from build123d import *

# Parameters (mm, degrees)
F2_DEPTH = 6
F3_R     = 1.5
F6_R     = 1.75
F7_DEPTH = 9
F8_R     = 3.5
F9_DEPTH = 5


with BuildPart() as f2:
    # F1 (on Front) → F2 (new body, symmetric)
    with BuildSketch(Plane.XZ):
        Polygon((-9, 0), (0, 0), (0, 70), (6, 70), (6, 66), (30, 66), (30, 79), (-9, 79), align=None)
    extrude(amount=F2_DEPTH, both=True)

    # F5: sweep along a path in F4
    with BuildLine(Plane.XZ) as f5_path:
        Line((-7.8191634321, 0), (-7.8191634321, 72.8191634321))
        ThreePointArc((-7.8191634321, 72.8191634321), (-6.3546973381, 76.3546973381), (-2.8191634321, 77.8191634321))
        Line((-2.8191634321, 77.8191634321), (30, 77.8191634321))
    # F3 (on face) → F5 (sweep, cut)
    with BuildSketch(Plane(origin=(0, 0, 0), x_dir=(1, 0, 0), z_dir=(0, 0, -1))):
        with Locations((-7.8191634321, 0)):
            Circle(F3_R)
    sweep(path=f5_path.line, mode=Mode.SUBTRACT)

    # F6 (on face) → F7 (cut, through all)
    with BuildSketch(Plane(origin=(-9, 0, 0), x_dir=(0, -1, 0), z_dir=(-1, 0, 0))):
        with Locations((0, 45.5)):
            Circle(F6_R)
        with Locations((0, 1)):
            Circle(F6_R)
    extrude(amount=-F7_DEPTH, mode=Mode.SUBTRACT)

    # F8 (on face) → F9 (cut)
    with BuildSketch(Plane(origin=(-9, 0, 0), x_dir=(0, -1, 0), z_dir=(-1, 0, 0))):
        with Locations((0, 45.5)):
            Circle(F8_R)
        with Locations((0, 1)):
            Circle(F8_R)
    extrude(amount=-F9_DEPTH, mode=Mode.SUBTRACT)


solid = f2.part
Geometry check sheet. Reference: the model listing, model coordinates, mm. A direction names the side the tool comes from. Give positions to 0.01 mm unless a question says otherwise; leave off trailing zeros. Write each loop counter-clockwise with the first axis right and the second up, starting at its lowest first coordinate (ties: lowest second). Pieces come first, ordered by that corner, then holes.
1) Thickness scan on line 1 (Y direction, x = -1.4, z = 1); line 2 (X direction, y = 0, z = 15.5); line 3 (Z direction, x = -5, y = 1.75). Record the ranges inside material, lowest first.
Values follow:
line 1: y = -6 to -1.75, 1.75 to 6
line 2: x = -6.32 to 0
line 3: z = 4.03 to 42.47, 48.53 to 79
2) Cross-section at A-A (z = 45.5). Record the boundary of the cut face in (x, y).
Values follow:
outline: (-9, -6) - (0, -6) - (0, -1.75) - (-4, -1.75) - (-4, -3.5) - (-9, -3.5) - close; (-9, 3.5) - (-4, 3.5) - (-4, 1.75) - (0, 1.75) - (0, 6) - (-9, 6) - close
3) Cross-section at B-B (y = 0). Record the boundary of the cut face in (x, z).
Values follow:
outline: (-9, 74.83) arc R6.5 cw to (-4.83, 79) - (-9, 79) - close; (-6.32, 4.5) - (-4, 4.5) - (-4, 2.75) - (0, 2.75) - (0, 43.75) - (-4, 43.75) - (-4, 42) - (-6.32, 42) - close; (-6.32, 49) - (-4, 49) - (-4, 47.25) - (0, 47.25) - (0, 70) - (6, 70) - (6, 66) - (30, 66) - (30, 76.32) - (-2.82, 76.32) arc R3.5 ccw to (-6.32, 72.82) - close
4) Set-up check for faces 1 (the face through (-6, -0.1, 4.5)), 2 (the face through (-6.32, -0.05, 60.91)), 3 (the face through (3, 0, 70)): record each of +Z, -Z, +X, -X, +Y, -Y from which the full face is reachable in a straight line by a thin tool's end or side.
Values follow:
face 1: -X
face 2: -Z
face 3: -Z, +Y, -Y
5) Release check for a two-part mould opening along Z. For faces 4 (the face through (-2.03, 0.38, 43.79)), 5 (the face through (-9, -1.4, 40.1)), 6 (the face through (10.8, -1.4, 79)) record: released by +Z, released by -Z, zero draft, split by the parting line, or undercut.
Values follow:
face 4: undercut
face 5: zero draft
face 6: released by +Z
6) Cross-section at C-C (x = -1.5). Record the boundary of the cut face in (y, z) (3 decimals), plus the area to 3 significant figures.
Values follow:
outline: (-6, 0) - (-1.436, 0) arc R1.75 cw (long way) to (1.436, 0) - (6, 0) - (6, 79) - (0.925, 79) arc R1.5 cw (long way) to (-0.925, 79) - (-6, 79) - close; hole circle Ø3.5 at (0, 45.5)
area: 924 mm2
7) Cross-section at D-D (x = 12). Record the boundary of the cut face in (y, z) (3 decimals), plus the area to 3 significant figures.
Values follow:
outline: (-6, 66) - (6, 66) - (6, 79) - (0.925, 79) arc R1.5 cw (long way) to (-0.925, 79) - (-6, 79) - close
area: 149 mm2
8) Go/stop test with flat-tipped pins: pin 1 Ø4.5 at (y, z) = (0, 1) entering from -X; pin 2 Ø2 at (x, y) = (6, -0.5) entering from -Z; pin 3 Ø3 at (y, z) = (-1.5, 11) entering from +X; pin 4 Ø2 at (y, z) = (0, 45.5) entering from -X. Record where each tip stops, or that it passes through.
Values follow:
pin 1: stops at x = -4
pin 2: stops at z = 66
pin 3: stops at x = 0
pin 4: passes through
